Design review of the part built by this model. Coordinates are the model's own, in mm. A direction names the side the tool comes from. Give positions to 0.01 mm unless a question says otherwise; leave off trailing zeros. Write each loop counter-clockwise with the first axis right and the second up, starting at its lowest first coordinate (ties: lowest second). Pieces come first, ordered by that corner, then holes. Notation, with made-up numbers: (74, 80) -> (133, 80) arc R14 ccw to (133, 92) -> close; hole circle Ø8 at (43.5, 74.5). An arc over 180 degrees is marked (long way). Answer as a JSON object with one key per item and string values.
```python
from build123d import *

# Parameters (mm, degrees)
SKETCH1_W             = 52
SKETCH1_H             = 256
BOSS_EXTRUDE1_DEPTH   = 6
M2_CLEARANCE_HOLE1_D  = 2.4
M2_CLEARANCE_HOLE2_D  = 2.4
M2_CLEARANCE_HOLE3_D  = 2.4
M2_CLEARANCE_HOLE4_D  = 2.4
M2_CLEARANCE_HOLE5_D  = 2.4
M2_CLEARANCE_HOLE6_D  = 2.4
M2_CLEARANCE_HOLE7_D  = 2.4
M2_CLEARANCE_HOLE8_D  = 2.4
M2_CLEARANCE_HOLE9_D  = 2.4
M2_CLEARANCE_HOLE10_D = 2.4
M2_CLEARANCE_HOLE11_D = 2.4
M2_CLEARANCE_HOLE12_D = 2.4
SKETCH26_W            = 36
SKETCH26_H            = 60
CUT_EXTRUDE2_DEPTH    = 6
SKETCH27_W            = 36
SKETCH27_H            = 60
CUT_EXTRUDE4_DEPTH    = 6


with BuildPart() as part:
    # Sketch1 → Boss-Extrude1 (new body)
    with BuildSketch(Plane(origin=(-157.1, 0, 0), x_dir=(0, 0, -1), z_dir=(1, 0, 0))):
        Rectangle(SKETCH1_W, SKETCH1_H)
    extrude(amount=BOSS_EXTRUDE1_DEPTH)

    # M2 Clearance Hole1 (through all)
    with Locations(Plane.ZY.offset(157.1)):
        with Locations((-4.5, 111.5)):
            Hole(M2_CLEARANCE_HOLE1_D / 2)

    # M2 Clearance Hole2 (through all)
    with Locations(Plane.ZY.offset(157.1)):
        with Locations((4.5, 111.5)):
            Hole(M2_CLEARANCE_HOLE2_D / 2)

    # M2 Clearance Hole3 (through all)
    with Locations(Plane.ZY.offset(157.1)):
        with Locations((-4.5, 120.5)):
            Hole(M2_CLEARANCE_HOLE3_D / 2)

    # M2 Clearance Hole4 (through all)
    with Locations(Plane.ZY.offset(157.1)):
        with Locations((4.5, 120.5)):
            Hole(M2_CLEARANCE_HOLE4_D / 2)

    # M2 Clearance Hole5 (through all)
    with Locations(Plane.ZY.offset(157.1)):
        with Locations((-4.5, -120.5)):
            Hole(M2_CLEARANCE_HOLE5_D / 2)

    # M2 Clearance Hole6 (through all)
    with Locations(Plane.ZY.offset(157.1)):
        with Locations((4.5, -120.5)):
            Hole(M2_CLEARANCE_HOLE6_D / 2)

    # M2 Clearance Hole7 (through all)
    with Locations(Plane.ZY.offset(157.1)):
        with Locations((-4.5, -111.5)):
            Hole(M2_CLEARANCE_HOLE7_D / 2)

    # M2 Clearance Hole8 (through all)
    with Locations(Plane.ZY.offset(157.1)):
        with Locations((4.5, -111.5)):
            Hole(M2_CLEARANCE_HOLE8_D / 2)

    # M2 Clearance Hole9 (through all)
    with Locations(Plane.ZY.offset(157.1)):
        with Locations((-15, -30)):
            Hole(M2_CLEARANCE_HOLE9_D / 2)

    # M2 Clearance Hole10 (through all)
    with Locations(Plane.ZY.offset(157.1)):
        with Locations((15, -30)):
            Hole(M2_CLEARANCE_HOLE10_D / 2)

    # M2 Clearance Hole11 (through all)
    with Locations(Plane.ZY.offset(157.1)):
        with Locations((-15, 30)):
            Hole(M2_CLEARANCE_HOLE11_D / 2)

    # M2 Clearance Hole12 (through all)
    with Locations(Plane.ZY.offset(157.1)):
        with Locations((15, 30)):
            Hole(M2_CLEARANCE_HOLE12_D / 2)

    # Sketch26 → Cut-Extrude2 (cut)
    with BuildSketch(Plane(origin=(-157.1, 0, 0), x_dir=(0, 0, -1), z_dir=(1, 0, 0))):
        with Locations((0, 70)):
            Rectangle(SKETCH26_W, SKETCH26_H)
    extrude(amount=CUT_EXTRUDE2_DEPTH, mode=Mode.SUBTRACT)

    # Sketch27 → Cut-Extrude4 (cut)
    with BuildSketch(Plane(origin=(-157.1, 0, 0), x_dir=(0, 0, -1), z_dir=(1, 0, 0))):
        with Locations((0, -70)):
            Rectangle(SKETCH27_W, SKETCH27_H)
    extrude(amount=CUT_EXTRUDE4_DEPTH, mode=Mode.SUBTRACT)


solid = part.part
```
(1) We need section A-A, the plane z = 0. State the section outline as (x, y) points.
Here are the results:
{"outline": "(-157.1, -128) -> (-151.1, -128) -> (-151.1, -100) -> (-157.1, -100) -> close; (-157.1, -40) -> (-151.1, -40) -> (-151.1, 40) -> (-157.1, 40) -> close; (-157.1, 100) -> (-151.1, 100) -> (-151.1, 128) -> (-157.1, 128) -> close"}
(2) We need section B-B, the plane y = -57. State the section outline as (x, z) points.
Here are the results:
{"outline": "(-157.1, -26) -> (-151.1, -26) -> (-151.1, -18) -> (-157.1, -18) -> close; (-157.1, 18) -> (-151.1, 18) -> (-151.1, 26) -> (-157.1, 26) -> close"}
(3) For faces 4 (the flat face through (-154, -2, -26)), 5 (the flat face through (-154, 70, 18)), list the 3-axis set-ups (+Z, -Z, +X, -X, +Y, -Y) from which the entire face can be reached by the end or side of a thin tool; tool diameter is ignored.
Here are the results:
{"face 4": "-Z, +X, -X, +Y, -Y", "face 5": "+X, -X"}
(4) Clearance check with a flat-ended pin moving along its axis: pin 1 (2 mm diameter, centred on y = -120.5, z = -4.5, fed in from -X). State where the tip first meets the part, or that it passes through.
Here are the results:
{"pin 1": "passes through"}
(5) The part is to be moulded in two halves that separate along X. For faces 1 (the flat face through (-151.1, 2, 0)), 2 (the flat face through (-157.1, 2, 0)), 3 (the flat face through (-154, 128, 0)), say which applies: +X half, -X half, draft (parallel to the pull), parting line (faces both ways), or undercut.
Here are the results:
{"face 1": "+X half", "face 2": "-X half", "face 3": "draft"}
(6) For line 1 along Z through (x, y) = (-155.4, 111.5); line 2 along Y through (x, z) = (-152.75, 6.5); line 3 along Y through (x, z) = (-153.55, 15), list the stretches that pass through material, from the lowest coordinate up.
Here are the results:
{"line 1": "z = -26 to -5.7, -3.3 to 3.3, 5.7 to 26", "line 2": "y = -128 to -100, -40 to 40, 100 to 128", "line 3": "y = -128 to -100, -40 to -31.2, -28.8 to 28.8, 31.2 to 40, 100 to 128"}
(7) We need section C-C, the plane x = -153.75. Give the number of separate pieces and of enclosed holes in the cut face, then the cut area to 3 significant figures.
Here are the results:
{"separate pieces": "1", "enclosed holes": "14", "area": "8,940 mm²"}
